from build123d import *

# Parameters (mm, degrees)
SKETCH1_W           = 79.75
SKETCH1_H           = 40
BOSS_EXTRUDE1_DEPTH = 3
SKETCH2_W           = 2.25
SKETCH2_H           = 10.5
CUT_EXTRUDE1_DEPTH  = 90.26960569
FILLET2_R           = 2.25
FILLET1_R           = 2.25
BOSS_EXTRUDE4_DEPTH = 3.7
SKETCH7_W           = 73.5
SKETCH7_H           = 35.5
OLED_RECESS_DEPTH   = 1.5
SKETCH9_R           = 1.7
CUT_EXTRUDE5_DEPTH  = 90.295870565


with BuildPart() as part:
    # Sketch1 → Boss-Extrude1 (new body)
    with BuildSketch(Plane.XY):
        with Locations((39.875, 20)):
            Rectangle(SKETCH1_W, SKETCH1_H)
    extrude(amount=BOSS_EXTRUDE1_DEPTH)

    # Sketch2 → Cut-Extrude1 (cut, through all)
    with BuildSketch(Plane.XY.offset(3)):
        with Locations((1.125, 20)):
            Rectangle(SKETCH2_W, SKETCH2_H)
    extrude(amount=-CUT_EXTRUDE1_DEPTH, mode=Mode.SUBTRACT)

    # Fillet2
    fillet2_edges = [part.edges().sort_by_distance(p)[0] for p in [
        (0, 14.75, 1.5),
        (0, 25.25, 1.5),
    ]]
    fillet(fillet2_edges, radius=FILLET2_R - 0.0001)  # a hair under: the kernel refuses the full size

    # Fillet1
    fillet1_edges = [part.edges().sort_by_distance(p)[0] for p in [
        (0, 40, 1.5),
        (0, 0, 1.5),
    ]]
    fillet(fillet1_edges, radius=FILLET1_R)

    # Sketch6 → Boss-Extrude4 (add)
    with BuildSketch(Plane.XY.offset(3)):
        with BuildLine():
            Line((1.25, 25.484435563), (1.25, 14.515564437))
            ThreePointArc((1.25, 14.515564437), (1.736443763, 14.69060722), (2.25, 14.75))
            Line((2.25, 14.75), (2.25, 25.25))
            ThreePointArc((2.25, 25.25), (1.736443763, 25.30939278), (1.25, 25.484435563))
        make_face()
    extrude(amount=-BOSS_EXTRUDE4_DEPTH)

    # Sketch7 → oled-recess (cut)
    with BuildSketch(Plane(origin=(0, 0, 0), x_dir=(-1, 0, 0), z_dir=(0, 0, -1))):
        with Locations((-40.75, 20)):
            Rectangle(SKETCH7_W, SKETCH7_H)
    extrude(amount=-OLED_RECESS_DEPTH, mode=Mode.SUBTRACT)

    # Sketch9 → Cut-Extrude5 (cut, through all)
    with BuildSketch(Plane.XY.offset(3)):
        with Locations((6, 34)):
            Circle(SKETCH9_R)
        with Locations((74, 34)):
            Circle(SKETCH9_R)
        with Locations((6, 6)):
            Circle(SKETCH9_R)
        with Locations((74, 6)):
            Circle(SKETCH9_R)
    extrude(amount=-CUT_EXTRUDE5_DEPTH, mode=Mode.SUBTRACT)


solid = part.part
Design review of the part built by this model. Coordinates are the model's own, in mm. A direction names the side the tool comes from. Round coordinates to 2 decimals unless told otherwise and drop trailing zeros. Loops run counter-clockwise (first coordinate to the right, second up) from the corner with the lowest first, then second, coordinate; pieces in that order, holes last. Notation, with made-up numbers: (85.25, 8.25) - (101.25, 8.25) arc R12 cw to (101.25, 15.25) - close; hole circle Ø6 at (75, 66.25). An arc over 180 degrees is marked (long way). One line per item, written item: value. Start each with the question number.
1) Draft analysis for pull direction Y (two halves, no side actions). For faces 1 (the cylindrical face through (0.68, 39.36, 1.52)), 2 (the flat face through (41, 20, 1.5)), 3 (the flat face through (0, 7, 1)), 4 (the cylindrical face through (72.3, 6.07, 2.26)), state which applies: +Y half, -Y half, draft (parallel to the pull), parting line (faces both ways), or undercut.
2) Insertion check: pin 1 Ø5 at (x, y) = (59.5, 8.5) entering from -Z; pin 2 Ø1.1 at (y, z) = (21, 1) entering from -X. Each pin has a flat end and moves straight along its axis. Give the tip position at first contact, or say it passes through.
3) To check wall thickness, follow L1, parallel to Y at x = 6, z = 2; L2, parallel to Y at x = 35, z = 0.6; L3, parallel to Z at x = 41.5, y = 25. State the ranges of each line that lie inside material, in increasing order. Write a range as from..to.
4) For faces 5 (the flat face through (1.25, 20, 1)), 6 (the flat face through (77.5, 20, 1)), 7 (the flat face through (39, 20, 3)), list the 3-axis set-ups (+Z, -Z, +X, -X, +Y, -Y) from which the entire face can be reached by the end or side of a thin tool; tool diameter is ignored.
5) Consider section B-B on y = 6. Give the boundary of the cut face in (x, z), then the cut area to 3 significant figures.
6) Consider section A-A on x = 74. Give the boundary of the cut face in (y, z).
7) Consider section D-D on x = 17.5. Give the boundary of the cut face in (y, z), then the cut area to 4 significant figures.
8) Consider section C-C on z = 2.2. Give the boundary of the cut face in (x, y), then the cut area to 3 significant figures.
Reported:
1. face 1: +Y half
1. face 2: undercut
1. face 3: draft
1. face 4: undercut
2. pin 1: stops at z = 1.5
2. pin 2: stops at x = 1.25
3. L1: y = 0..4.3, 7.7..32.3, 35.7..40
3. L2: y = 0..2.25, 37.75..40
3. L3: z = 1.5..3
4. face 5: +Z, -Z, -X
4. face 6: -Z
4. face 7: +Z, +X, -X, +Y, -Y
5. outline: (0, 0) - (4, 0) - (4, 1.5) - (4.3, 1.5) - (4.3, 3) - (0, 3) - close; (7.7, 1.5) - (72.3, 1.5) - (72.3, 3) - (7.7, 3) - close; (75.7, 1.5) - (77.5, 1.5) - (77.5, 0) - (79.75, 0) - (79.75, 3) - (75.7, 3) - close
5. area: 119 mm^2
6. outline: (0, 0) - (2.25, 0) - (2.25, 1.5) - (4.3, 1.5) - (4.3, 3) - (0, 3) - close; (7.7, 1.5) - (32.3, 1.5) - (32.3, 3) - (7.7, 3) - close; (35.7, 1.5) - (37.75, 1.5) - (37.75, 0) - (40, 0) - (40, 3) - (35.7, 3) - close
7. outline: (0, 0) - (2.25, 0) - (2.25, 1.5) - (37.75, 1.5) - (37.75, 0) - (40, 0) - (40, 3) - (0, 3) - close
7. area: 66.75 mm^2
8. outline: (0, 2.25) arc R2.25 ccw to (2.25, 0) - (79.75, 0) - (79.75, 40) - (2.25, 40) arc R2.25 ccw to (0, 37.75) - (0, 27.5) arc R2.25 ccw to (1.25, 25.48) - (1.25, 14.52) arc R2.25 ccw to (0, 12.5) - close; hole circle Ø3.4 at (6, 6); hole circle Ø3.4 at (6, 34); hole circle Ø3.4 at (74, 6); hole circle Ø3.4 at (74, 34)
8. area: 3,140 mm^2
